Autodesk Inventor part; units mm, degrees
ref_plane "YZ Plane" through (0, 0, 0) normal (1, 0, 0) x (0, 1, 0)
ref_plane "XZ Plane" through (0, 0, 0) normal (0, 1, 0) x (-1, 0, 0)
ref_plane "XY Plane" through (0, 0, 0) normal (0, 0, 1) x (1, 0, 0)
sketch "Sketch1" plane through (0, 0, 0) normal (0, 1, 0) x (-1, 0, 0)
  line L0 (0, 0) -> (0, 12.7)
  arc A0 (0, 12.7) -> (-64.77, 77.47) centre (-64.77, 12.7) ccw
  line L1 (0, 0) -> (38.1, 0)
  line L2 (-64.77, 77.47) -> (-152.4, 77.47)
  line L3 (-152.4, 77.47) -> (-152.4, 83.82)
  line L4 (-152.4, 83.82) -> (-64.77, 83.82)
  arc A1 (6.35, 12.7) -> (-64.77, 83.82) centre (-64.77, 12.7) ccw
  arc A2 (38.1, 0) -> (6.35, 12.7) centre (19.685, 0) ccw
  line L5 (81.359, 0) -> (-191.3598, 0)
  dimension "d0" = 12.7
  dimension "d4" = 152.4
  dimension "d5" = 77.47
  dimension "d6" = 6.35
  dimension "d7" = 12.7
  dimension "d9" = 38.1
revolve "Revolution1" add sketch "Sketch1" angle 360 about axis through (-10, 0, 0) along (1, 0, 0)
sketch "Sketch3" plane through (0, 0, 0) normal (0, 1, 0) x (-1, 0, 0)
  line L0 (-99.1769, -83.82) -> (-99.1769, -49.0516)
  line L1 (-99.1769, 83.82) -> (-99.1769, 47.9401)
  line L2 (-152.4, -83.82) -> (-152.4, 83.82)
  line L3 (-99.1769, -49.0516) -> (-124.5769, -49.0516)
  line L4 (-99.1769, 47.9401) -> (-124.5769, 47.9401)
  line L5 (-152.4, -83.82) -> (-64.77, -83.82)
  line L6 (-152.4, 83.82) -> (-64.77, 83.82)
  line L7 (-99.1769, -83.82) -> (-152.4, -83.82)
  line L8 (-152.4, 83.82) -> (-99.1769, 83.82)
  line L9 (-152.4, -83.82) -> (-152.4, 83.82)
  line L10 (-151.13, -9.525) -> (-151.13, 9.525)
  line L11 (76.2, 0) -> (-190.5, 0)
  arc A0 (-151.13, -9.525) -> (-124.5769, -49.0516) centre (-108.4341, -9.525) ccw
  arc A1 (-124.5769, 47.9401) -> (-151.13, 9.525) centre (-110.0654, 9.525) ccw
  point P0 (0, 0)
  point P1 (-152.4, 0)
  point P2 (-151.13, 0)
  dimension "d14" = 25.4
  dimension "d15" = 25.4
  dimension "d18" = 34.7684
  dimension "d22" = 53.2231
  dimension "d23" = 35.8799
  dimension "d26" = 19.05
  dimension "d27" = 1.27
extrude "Extrusion1" cut sketch "Sketch3" along normal through all both and the other way through all
sketch "Sketch4" plane through (151.13, -83.277, -9.525) normal (1, 0, 0) x (0, 0, -1)
  arc A0 (-19.05, 6.3948) -> (0, 6.3948) centre (-9.525, 83.277) ccw
  arc A1 (-19.05, 0) -> (0, 0) centre (-9.525, 83.277) ccw
  circle A2 centre (-9.525, 1.994) radius 6.35
  arc A3 (0, 160.1593) -> (-19.05, 160.1593) centre (-9.525, 83.277) ccw
  arc A4 (0, 166.5541) -> (-19.05, 166.5541) centre (-9.525, 83.277) ccw
  circle A5 centre (-9.525, 164.557) radius 6.35
  point P0 (-9.525, 160.747)
  dimension "d28" = 12.7
  dimension "d30" = 81.2831
  dimension "d31" = 12.7
  dimension "d32" = 81.28
extrude "Extrusion2" add sketch "Sketch4" along normal blind 76.2
properties part number "DMJ_hat"
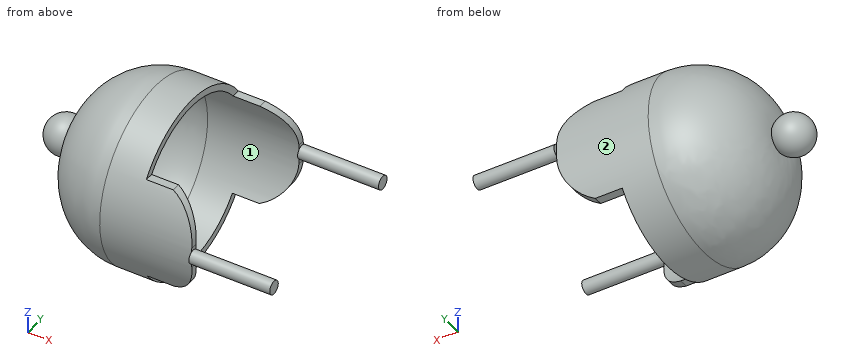
Can you work these out from the model? Positions are in its coordinate system, mm. Face numbers are marked on the shaded views. Coordinates: 2 decimals unless noted, no trailing zeros. Write each loop counter-clockwise with the first axis right and the second up, starting at its lowest first coordinate (ties: lowest second). Pieces come first, ordered by that corner, then holes. Notation, with made-up numbers: (56.25, 22) - (75.25, 22) arc R17 ccw to (75.25, 29) - close; hole circle Ø3 at (0.5, 61.5). An arc over 180 degrees is marked (long way). Return JSON: item names as keys, results as strings. Group by question number.
Item 1: Please list where these lines run through material, in increasing order: probe 1 along Y at (x, z) = (73, -0.5); probe 2 along Y at (x, z) = (125, -10).
Item 2: If we section it at A-A (x = 112): Write out the boundary of the cut face in (y, z).
Item 3: If we section it at B-B (x = 158): Write out the boundary of the cut face in (y, z).
Item 4: We'd pull the mould along Z, two halves only. Please class the marked faces 1 and 2: pulls with the +Z half, pulls with the -Z half, needs draft (parallel to the pull), parting line crosses it, or undercut.
Item 5: I'm going to push flat-ended pins straight in: pin 1 Ø12 at (y, z) = (37, 66.5) entering from +X; pin 2 Ø1.4 at (y, z) = (79, 7) entering from +X; pin 3 Ø18 at (y, z) = (12.5, 61) entering from +X; pin 4 Ø5 at (y, z) = (-80.5, -8.5) entering from +X. Where does each tip first touch, or does it pass through?
Return value:
{
 "1": {"probe 1": "y = -83.82 to -77.47, 77.47 to 83.82", "probe 2": "y = -83.22 to -76.82, 76.82 to 83.22"},
 "2": {"outline": "(-68.76, 47.94) arc R83.82 ccw to (-67.97, -49.05) - (-59.96, -49.05) arc R77.47 cw to (-60.86, 47.94) - close; (59.96, -49.05) - (67.97, -49.05) arc R83.82 ccw to (68.76, 47.94) - (60.86, 47.94) arc R77.47 cw to start"},
 "3": {"outline": "circle Ø12.7 at (-81.28, 0); circle Ø12.7 at (81.28, 0)"},
 "4": {"face 1": "undercut", "face 2": "parting line crosses it"},
 "5": {"pin 1": "stops at x = 99.18", "pin 2": "stops at x = 151.13", "pin 3": "stops at x = 37.11", "pin 4": "stops at x = 227.33"}
}
